Could you check a few things on this model? Use its own coordinates, in mm. A direction names the side the tool comes from. Round coordinates to 2 decimals unless told otherwise and drop trailing zeros. Order: outer loops, then holes, each group sorted by start corner. A loop starts at its lowest first (then second) coordinate and runs counter-clockwise, first axis right, second up. Notation, with made-up numbers: (0, 39) - (50, 39) arc R18 ccw to (50, 51) - close; hole circle Ø9 at (-28, 37). An arc over 180 degrees is marked (long way). Use one line per item in the form item = value.
from build123d import *

# Parameters (mm, degrees)
F0_R     = 45
F0_R_2   = 13.1526649771
F1_DEPTH = 3.5
F2_R     = 3
F3_R     = 25
F3_R_2   = 13.1526649771
F4_DEPTH = 12
F5_R     = 2


with BuildPart() as f1:
    # F0 (on Front) → F1 (new body)
    with BuildSketch(Plane.XZ):
        Circle(F0_R)
        Circle(F0_R_2, mode=Mode.SUBTRACT)
    extrude(amount=F1_DEPTH)

    # F2
    f2_edges = [f1.edges().sort_by_distance(p)[0] for p in [
        (-45, -3.5, 0),
    ]]
    fillet(f2_edges, radius=F2_R)

    # F3 (on face) → F4 (join)
    with BuildSketch(Plane.XZ.offset(3.5)):
        Circle(F3_R)
        Circle(F3_R_2, mode=Mode.SUBTRACT)
    extrude(amount=F4_DEPTH)

    # F5
    f5_edges = [f1.edges().sort_by_distance(p)[0] for p in [
        (-13.152665, -15.5, 0),
        (-25, -15.5, 0),
    ]]
    fillet(f5_edges, radius=F5_R)


solid = f1.part
Item 1: For faces 1 (the face through (18, -3.5, -18)), 2 (the face through (20.765, -0.246, -39.923)), which set-ups out of +Z, -Z, +X, -X, +Y, -Y let a thin tool reach every point of the face, with its end or its side?
Found:
face_1 = -Y
face_2 = +Y, -Y
Item 2: I need wall thicknesses on L1, parallel to Z at x = 0, y = -8.75; L2, parallel to Y at x = -26.5, z = 1.5; L3, parallel to Z at x = 4.5, y = -4. Which ranges of each line are inside material? Lowest first, please.
Found:
L1 = -25 to -13.15, 13.15 to 25
L2 = -3.5 to 0
L3 = -24.59 to -12.36, 12.36 to 24.59
Item 3: Imagine slicing it at C-C on y = -9. Please give me the cut outline in (x, z).
Found:
outline = circle Ø50 at (0, 0); hole circle Ø26.31 at (0, 0)
Item 4: Will these pins go through, and if not, where does the flat tip stop? P1, Ø2, axis at x = -2, y = -8, coming from the +Z side; P2, Ø8, axis at y = -10.5, z = -9.5, coming from the -X side; P3, Ø1, axis at x = 30, z = 33.5, coming from the -Y side.
Found:
P1 = 24.98
P2 = -24.39
P3 = -2.2
Item 5: Imagine slicing it at B-B on x = 0. Please give me the cut outline in (y, z), plus the area to 3 significant figures.
Found:
outline = (-15.5, -23) arc R2 ccw to (-13.5, -25) - (-3.5, -25) - (-3.5, -42) arc R3 ccw to (-0.5, -45) - (0, -45) - (0, -13.15) - (-13.5, -13.15) arc R2 ccw to (-15.5, -15.15) - close; (-15.5, 15.15) arc R2 ccw to (-13.5, 13.15) - (0, 13.15) - (0, 45) - (-0.5, 45) arc R3 ccw to (-3.5, 42) - (-3.5, 25) - (-13.5, 25) arc R2 ccw to (-15.5, 23) - close
area = 500 mm2
Item 6: If we mould it in two halves opening along Z, with no side actions, what happens to faces 3 (the face through (9, 0, 11)), 4 (the face through (12.15, -6.66, -5.04)), 5 (the face through (23.846, -8.43, 7.509))? For each: released by +Z, released by -Z, zero draft, split by the parting line, or undercut.
Found:
face_3 = zero draft
face_4 = undercut
face_5 = split by the parting line
Item 7: Imagine slicing it at A-A on z = 0. Please give me the cut outline in (x, y).
Found:
outline = (-45, -0.5) arc R3 ccw to (-42, -3.5) - (-25, -3.5) - (-25, -13.5) arc R2 ccw to (-23, -15.5) - (-15.15, -15.5) arc R2 ccw to (-13.15, -13.5) - (-13.15, 0) - (-45, 0) - close; (13.15, -13.5) arc R2 ccw to (15.15, -15.5) - (23, -15.5) arc R2 ccw to (25, -13.5) - (25, -3.5) - (42, -3.5) arc R3 ccw to (45, -0.5) - (45, 0) - (13.15, 0) - close
